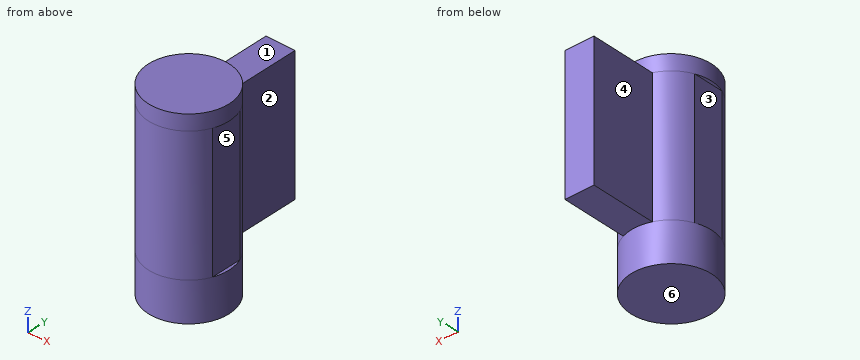
```python
from build123d import *

# Parameters (mm, degrees)
F1_DEPTH = 26.04
F2_R     = 7.81
F3_DEPTH = 3
F4_R     = 7.81
F5_DEPTH = 7.65


with BuildPart() as f1:
    # F0 (on Top) → F1 (new body)
    with BuildSketch(Plane.XY):
        with BuildLine():
            Line((-2.81, 20), (-2.81, 7.286975))
            ThreePointArc((-2.81, 7.286975), (-5.449661, 5.594398), (-7.210832, 3))
            Line((-7.210832, 3), (-7.210832, 0))
            Line((-7.210832, 0), (7.210832, 0))
            Line((7.210832, 0), (7.210832, 3))
            ThreePointArc((7.210832, 3), (5.449661, 5.594398), (2.81, 7.286975))
            Line((2.81, 7.286975), (2.81, 20))
            Line((2.81, 20), (-2.81, 20))
        make_face()
        with BuildLine():
            Line((7.210832, 0), (-7.210832, 0))
            Line((-7.210832, 0), (-7.210832, -3))
            ThreePointArc((-7.210832, -3), (0, -7.81), (7.210832, -3))
            Line((7.210832, -3), (7.210832, 0))
        make_face()
    extrude(amount=F1_DEPTH)

    # F2 (on face) → F3 (join)
    with BuildSketch(Plane.XY.offset(26.04)):
        Circle(F2_R)
    extrude(amount=F3_DEPTH)

    # F4 (on face) → F5 (join)
    with BuildSketch(Plane(origin=(0, 0, 0), x_dir=(1, 0, 0), z_dir=(0, 0, -1))):
        Circle(F4_R)
    extrude(amount=F5_DEPTH)


solid = f1.part
```
Can you work these out from the model? Positions are in its coordinate system, mm. Face numbers are marked on the shaded views. A direction names the side the tool comes from. Give positions to 0.01 mm unless a question says otherwise; leave off trailing zeros. Loops run counter-clockwise (first coordinate to the right, second up) from the corner with the lowest first, then second, coordinate; pieces in that order, holes last. Notation, with made-up numbers: M -19,52 L 14,52 A12 cw 14,59 Z; hole C 20.5,33 d3. An arc over 180 degrees is marked long. Use one line per item in the form item = value. Start each with the question number.
(1) On a 3-axis mill with a long thin cutter (end or side, diameter ignored), from which of +Z, -Z, +X, -X, +Y, -Y can I reach the whole of each face in a straight line? I mean the marked faces 4, 5 and 6. Say none if no direction works.
(2) Please list where these lines run through material, in increasing order: line 1 (Y direction, x = 0.25, z = 14.5); line 2 (X direction, y = 2.25, z = 5); line 3 (X direction, y = 18.75, z = 17.5).
(3) I want a section at D-D, the plane y = 9. Write out the boundary of the cut face in (x, z), and give its area (3 significant figures).
(4) Thinking about a two-plate mould opening in Z: for the marked faces 1, 2 and 3, which applies, released by +Z, released by -Z, zero draft, split by the parting line, or undercut?
(5) I want a section at C-C, the plane y = 0. Write out the boundary of the cut face in (x, z).
(6) I want a section at B-B, the plane x = 0. Write out the boundary of the cut face in (y, z).
(7) I want a section at A-A, the plane z = 13. Write out the boundary of the cut face in (x, y).
(8) I'm going to push flat-ended pins straight in: P1, Ø3, axis at y = -2, z = 11, coming from the +X side; P2, Ø2, axis at x = -3, z = 24.5, coming from the -Y side; P3, Ø3, axis at x = -1, y = 13, coming from the +Z side. Where does each tip first touch, or does it pass through?
Worked out:
q1.face_4 = +Z, -Z, -X, +Y
q1.face_5 = +X, +Y, -Y
q1.face_6 = -Z, +X, -X, +Y, -Y
q2.line_1 = -7.81 to 20
q2.line_2 = -7.21 to 7.21
q2.line_3 = -2.81 to 2.81
q3.outline = M -2.81,0 L 2.81,0 L 2.81,26.04 L -2.81,26.04 Z
q3.area = 146 mm²
q4.face_1 = released by +Z
q4.face_2 = zero draft
q4.face_3 = undercut
q5.outline = M -7.81,-7.65 L 7.81,-7.65 L 7.81,0 L 7.21,0 L 7.21,26.04 L 7.81,26.04 L 7.81,29.04 L -7.81,29.04 L -7.81,26.04 L -7.21,26.04 L -7.21,0 L -7.81,0 Z
q6.outline = M -7.81,-7.65 L 7.81,-7.65 L 7.81,0 L 20,0 L 20,26.04 L 7.81,26.04 L 7.81,29.04 L -7.81,29.04 Z
q7.outline = M -7.21,-3 A7.81 ccw 7.21,-3 L 7.21,3 A7.81 ccw 2.81,7.29 L 2.81,20 L -2.81,20 L -2.81,7.29 A7.81 ccw -7.21,3 Z
q8.P1 = 7.21
q8.P2 = -7.55
q8.P3 = 26.04
